Work out the finished part from the listing and answer in its coordinate system (mm). A direction names the side the tool comes from. Coordinates: 2 decimals unless noted, no trailing zeros. Loops run counter-clockwise (first coordinate to the right, second up) from the corner with the lowest first, then second, coordinate; pieces in that order, holes last. Notation, with made-up numbers: (2.5, 20) - (42.5, 20) arc R30 ccw to (42.5, 50) - close; hole circle Ø2 at (4, 18.25). An arc over 180 degrees is marked (long way). Write each question's results on one line, items separated by ' | '. Start each with the question number.
Item 1: Section D-D, the plane x = 47.5 is taken. Write down the section's boundary in (y, z).
Item 2: Each of these flat-tipped pins is pushed along its axis until it touches: pin 1 Ø11 at (y, z) = (-35, 4.5) entering from +X; pin 2 Ø3 at (x, y) = (10, -3.5) entering from +Z; pin 3 Ø11 at (x, z) = (43.5, 6) entering from -Y; pin 4 Ø3 at (y, z) = (-40.5, 13) entering from -X. Where does it stop, or does it pass through?
Item 3: Section B-B, the plane y = -6.5 is taken. Write down the section's boundary in (x, z), plus the area to 3 significant figures.
Item 4: Section C-C, the plane x = 18 is taken. Write down the section's boundary in (y, z).
Item 5: A tool of negligible diameter and unlimited length cuts with its end or side. For faces 1 (the face through (40, -20, 5)), 2 (the face through (23, -25, 10)), 3 (the face through (10, -5, 30)), from which of +Z, -Z, +X, -X, +Y, -Y can it reach the whole face along a straight path? Write none if from no direction.
Item 6: For a pull along X with two mould halves and no side action, classify faces 4 (the face through (26.99, -47.15, 4.93)), 5 (the face through (10, -50, 5)), 6 (the face through (35, -5, 20)), 7 (the face through (20, -5, 25)) as +X half, -X half, draft (parallel to the pull), parting line (faces both ways), or undercut.
Item 7: Consider probe 1 along Z at (x, y) = (14.5, -19.5); probe 2 along Y at (x, z) = (52, 30.5); probe 3 along Z at (x, y) = (3.5, -5.5). Determine where each line is inside the solid, lowest interval first. Write a range as [from, to].
Item 8: Section A-A, the plane z = 7 is taken. Write down the section's boundary in (x, y), plus the area to 3 significant figures.
from build123d import *

# Parameters (mm, degrees)
F1_DEPTH = 10
F3_DEPTH = 10


# Not quite as in the source:
# - a feature names something its author has since deleted; it is built from what else it names


with BuildPart() as f1:
    # F0 (on Top) → F1 (new body)
    with BuildSketch(Plane.XY):
        with BuildLine():
            Line((60, 0), (20, 0))
            Line((20, 0), (0, 0))
            Line((0, 0), (0, -50))
            Line((0, -50), (20, -50))
            ThreePointArc((20, -50), (27.0710678119, -47.0710678119), (30, -40))
            Line((30, -40), (30, -20))
            Line((30, -20), (50, -20))
            ThreePointArc((50, -20), (57.0710678119, -17.0710678119), (60, -10))
            Line((60, -10), (60, 0))
        make_face()
    extrude(amount=F1_DEPTH)

    # F2 (on Front) → F3 (join)
    with BuildSketch(Plane.XZ):
        with BuildLine():
            Line((0, 30), (0, 10))
            Line((0, 10), (60, 10))
            Line((60, 10), (60, 40))
            ThreePointArc((60, 40), (57.0710678119, 47.0710678119), (50, 50))
            Line((50, 50), (50, 20))
            Line((50, 20), (20, 20))
            Line((20, 20), (20, 30))
            Line((20, 30), (0, 30))
        make_face()
    extrude(amount=F3_DEPTH)


solid = f1.part
Answer key:
1) outline: (-20, 0) - (0, 0) - (0, 20) - (-10, 20) - (-10, 10) - (-20, 10) - close
2) pin 1: stops at x = 30 | pin 2: stops at z = 30 | pin 3: stops at y = -20 | pin 4: passes through
3) outline: (0, 0) - (60, 0) - (60, 40) arc R10 ccw to (50, 50) - (50, 20) - (20, 20) - (20, 30) - (0, 30) - close | area: 1,680 mm^2
4) outline: (-50, 0) - (0, 0) - (0, 30) - (-10, 30) - (-10, 10) - (-50, 10) - close
5) face 1: +Z, -Z, +X, -Y | face 2: +Z, +X, -X, -Y | face 3: +Z, -X, +Y, -Y
6) face 4: +X half | face 5: draft | face 6: undercut | face 7: undercut
7) probe 1: z = [0, 10] | probe 2: y = [-10, 0] | probe 3: z = [0, 30]
8) outline: (0, -50) - (20, -50) arc R10 ccw to (30, -40) - (30, -20) - (50, -20) arc R10 ccw to (60, -10) - (60, 0) - (0, 0) - close | area: 2,060 mm^2
